Verification items for the finished model (mm, model axes). Face numbers are marked on the shaded views. Coordinates: 2 decimals unless noted, no trailing zeros. Loops run counter-clockwise (first coordinate to the right, second up) from the corner with the lowest first, then second, coordinate; pieces in that order, holes last. Notation, with made-up numbers: (-22.5, 38.25) - (7.5, 38.25) arc R28 cw to (7.5, 66.25) - close; hole circle Ø7 at (36.5, 88.25). An arc over 180 degrees is marked (long way). Answer as CSV lines item,"result". Start each with the question number.
1. Cross-section at A-A (z = -27.5). Enter the section's corners in (x, y), plus the area to 3 significant figures.
2. Gauge pin test, flat ends, axial feed: P1, Ø23.5, axis at y = 25.5, z = 74, coming from the -X side; P2, Ø10, axis at x = 22, z = 2.5, coming from the +Y side; P3, Ø1.5, axis at y = -27.5, z = 47.5, coming from the -X side; P4, Ø2, axis at x = 70, y = -9, coming from the -Z side. Record the tip position at first contact, or that the pin passes through.
3. Material ranges on line 1 (Y direction, x = 10.5, z = 61.5); line 2 (Y direction, x = 80, z = -5); line 3 (X direction, y = 48.5, z = 33), recorded low to high. Write a range as [from, to].
4. Cross-section at C-C (z = 2). Enter the section's corners in (x, y), plus the area to 3 significant figures.
5. Cross-section at B-B (x = 10). Enter the section's corners in (y, z), plus the area to 3 significant figures.
6. Cross-section at D-D (x = 61). Enter the section's corners in (y, z), plus the area to 3 significant figures.
7. Release check for a two-part mould opening along X. For the marked faces 1 and 2 record: pulls with the +X half, pulls with the -X half, needs draft (parallel to the pull), parting line crosses it, or undercut.
```python
from build123d import *

# Parameters (mm, degrees)
REVOLVE1_ANGLE      = 180
CUT_EXTRUDE1_DEPTH  = 172.464281995
CUT_EXTRUDE2_DEPTH  = 147.710676959
CHAMFER1_SIZE       = 5
SHELL1_T            = -2
BOSS_EXTRUDE1_DEPTH = 2


with BuildPart() as part:
    # Sketch1 → Revolve1 (revolve)
    with BuildSketch(Plane(origin=(0, 0, 0), x_dir=(0, 0, -1), z_dir=(1, 0, 0))):
        with BuildLine():
            Line((0, -55), (0, 55))
            Line((0, 55), (-75, 55))
            ThreePointArc((-75, 55), (-93.005376189, 0), (-75, -55))
            Line((-75, -55), (0, -55))
        make_face()
    revolve(axis=Axis((0, -55, 0), (0, 1, 0)), revolution_arc=REVOLVE1_ANGLE)

    # Sketch2 → Cut-Extrude1 (cut, through all)
    with BuildSketch(Plane.XZ.offset(55)):
        Polygon((0, 0), (0, 40), (12.287280664, 48.603646545), (12.287280664, 112.259604339), (-94.581934809, 112.259604339), (-94.581934809, -108.477643872), (97.057130945, -108.477643872), (97.057130945, -61.701791886), (17.67766953, 17.67766953), align=None)
    extrude(amount=-CUT_EXTRUDE1_DEPTH, mode=Mode.SUBTRACT)

    # Sketch3 → Cut-Extrude2 (cut, through all)
    with BuildSketch(Plane(origin=(100, 0, 0), x_dir=(0, 0, -1), z_dir=(1, 0, 0))):
        Polygon((-60, -15), (-60, 15), (45.666627767, 30), (45.666627767, -30), align=None)
    extrude(amount=-CUT_EXTRUDE2_DEPTH, mode=Mode.SUBTRACT)

    # Chamfer1
    # the kernel refuses this chamfer: 5, 4.450979534 mm, written as the material it takes off along each edge
    with BuildSketch(Plane(origin=(12.287280664, 0, 0), x_dir=(0, 0.7023997796774999, 0.7117826560889214), z_dir=(0, 0.7117826560889214, -0.7023997796774999))) as chamfer1_piece_1:
        with BuildLine():
            Line((92.190144451 - CHAMFER1_SIZE, 0), (91.510568486, 4.320424035))
            ThreePointArc((91.510568486, 4.320424035), (91.866596239, 2.222319448), (92.190144451, 0))
            Line((92.190144451, 0), (92.190144451 - CHAMFER1_SIZE, 0))
        make_face()
    revolve(axis=Axis((12.287280664, 0, 0), (1, 0, 0)), revolution_arc=89.239714317, mode=Mode.SUBTRACT)

    # Shell1
    shell1_openings = [part.faces().sort_by_distance(p)[0] for p in [
        (0, -37.799975499, 20.551470825),
        (44.318791783, -39.564539913, -8.963452724),
        (12.287280664, 0, 66.554150501),
        (8.951756718, -38.623299359, 8.951756718),
        (6.176749303, -36.112578818, 44.325006424),
        (8.951756718, 38.623299359, 8.951756718),
        (44.318791783, 39.564539913, -8.963452724),
        (6.176749303, 36.112578818, 44.325006424),
        (0, 37.799975499, 20.551470825),
        (41.411625019, 0, 60),
        (50.400096072, 20.67683416, 20.009871862),
        (50.400096072, -20.67683416, 20.009871862),
    ]]
    offset(amount=SHELL1_T, openings=shell1_openings)

    # Sketch4 → Boss-Extrude1 (add)
    with BuildSketch(Plane.XZ.offset(55)):
        Polygon((12.287280664, 67.654425497), (0, 55.367144833), (0, 40), (12.287280664, 48.603646545), align=None)
    boss_extrude1 = extrude(amount=-BOSS_EXTRUDE1_DEPTH)

    # Mirror1: Boss-Extrude1 across plane
    add(boss_extrude1.mirror(Plane.ZX))


solid = part.part
```
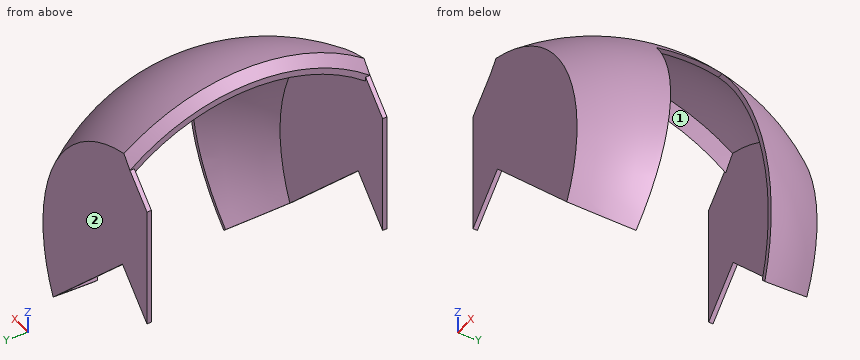
Values follow:
1,outline,"(62.86, -55) - (69.78, -55) arc R88.85 ccw to (84.51, -27.42) - (82.3, -27.42) arc R86.75 cw to (68.68, -53) - (62.86, -53) - close; (62.86, 53) - (68.68, 53) arc R86.75 cw to (82.3, 27.42) - (84.51, 27.42) arc R88.85 ccw to (69.78, 55) - (62.86, 55) - close"
1,area,"152 mm²"
2,P1,"stops at x = 12.29"
2,P2,"passes through"
2,P3,"stops at x = 72.02"
2,P4,"stops at z = 60"
3,line 1,"y = [-55, -53], [53, 55]"
3,line 2,"y = [-47.17, -43.09], [43.09, 47.17]"
3,line 3,"x = [69.58, 72.17]"
4,outline,"(0, -55) - (2, -55) - (2, -53) - (0, -53) - close; (0, 53) - (2, 53) - (2, 55) - (0, 55) - close; (33.36, -55) - (74.97, -55) arc R92.98 ccw to (90.03, -23.23) - (87.97, -23.23) arc R90.98 cw to (73.95, -53) - (33.36, -53) - close; (33.36, 53) - (73.95, 53) arc R90.98 cw to (87.97, 23.23) - (90.03, 23.23) arc R92.98 ccw to (74.97, 55) - (33.36, 55) - close"
4,area,"309 mm²"
5,outline,"(-55, 10) - (-53, 10) - (-53, 65.37) - (-55, 65.37) - close; (53, 10) - (55, 10) - (55, 65.37) - (53, 65.37) - close"
5,area,"221 mm²"
6,outline,"(-55, -25.64) - (-53, -25.64) - (-53, 41.86) arc R67.54 cw to (53, 41.86) - (53, -25.64) - (55, -25.64) - (55, 43.63) arc R70.21 ccw to (-55, 43.63) - close"
6,area,"605 mm²"
7,face 1,"undercut"
7,face 2,"needs draft"
